Part model, mm, in its own coordinate system. Face numbers are marked on the shaded views. Coordinates: 2 decimals unless noted, no trailing zeros. Order: outer loops, then holes, each group sorted by start corner. A loop starts at its lowest first (then second) coordinate and runs counter-clockwise, first axis right, second up.
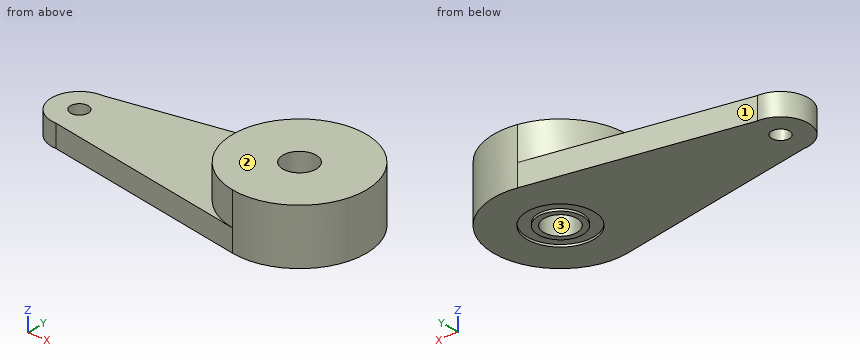
from build123d import *

# Parameters (mm, degrees)
F0_R     = 1.5
F1_DEPTH = 5
F0_R_2   = 0.8
F2_DEPTH = 2
F3_R     = 3
F3_R_2   = 2
F4_DEPTH = 0.2


with BuildPart() as f1:
    # F0 (on Top) → F1 (new body)
    with BuildSketch(Plane.XY):
        with BuildLine():
            ThreePointArc((-1.0798815668, -5.9020213319), (3.8419207826, -4.6086489018), (6, 0))
            ThreePointArc((6, 0), (3.8419207985, 4.6086488886), (-1.0798815261, 5.9020213393))
            ThreePointArc((-1.0798815261, 5.9020213393), (-6, 2.07e-08), (-1.0798815668, -5.9020213319))
        make_face()
        Circle(F0_R, mode=Mode.SUBTRACT)
    extrude(amount=F1_DEPTH)

    # F0 (on Top) → F2 (join)
    with BuildSketch(Plane.XY):
        with BuildLine():
            ThreePointArc((-1.0798815668, -5.9020213319), (-6, 2.07e-08), (-1.0798815261, 5.9020213393))
            Line((-1.0798815261, 5.9020213393), (-19.6734044441, 2.5))
            ThreePointArc((-19.6734044441, 2.5), (-17.9056374912, 1.767766953), (-17.1734044441, 0))
            ThreePointArc((-17.1734044441, 0), (-17.9056374912, -1.767766953), (-19.6734044441, -2.5))
            Line((-19.6734044441, -2.5), (-1.0798815668, -5.9020213319))
        make_face()
        with BuildLine():
            ThreePointArc((-17.1734044441, 0), (-17.9056374912, 1.767766953), (-19.6734044441, 2.5))
            ThreePointArc((-19.6734044441, 2.5), (-22.1734044441, 0), (-19.6734044441, -2.5))
            ThreePointArc((-19.6734044441, -2.5), (-17.9056374912, -1.767766953), (-17.1734044441, 0))
        make_face()
        with Locations((-19.6734044441, 0)):
            Circle(F0_R_2, mode=Mode.SUBTRACT)
    extrude(amount=F2_DEPTH)

    # F3 (on face) → F4 (cut)
    with BuildSketch(Plane(origin=(0, 0, 0), x_dir=(1, 0, 0), z_dir=(0, 0, -1))):
        Circle(F3_R)
        Circle(F3_R_2, mode=Mode.SUBTRACT)
    extrude(amount=-F4_DEPTH, mode=Mode.SUBTRACT)


solid = f1.part
Q1. Wall check: line 1 along Y through (x, z) = (0, 0.1); line 2 along Y through (x, z) = (0, 1.25); line 3 along Z through (x, y) = (-7, 1.25). Give the ranges that are in metal, low to high.
Results list:
line 1: y = -6 to -3, -2 to -1.5, 1.5 to 2, 3 to 6
line 2: y = -6 to -1.5, 1.5 to 6
line 3: z = 0 to 2
Q2. Cut at C-C on y = 0. Write the cut outline in (x, z), and give its area (3 significant figures).
Results list:
outline: (-22.17, 0) - (-20.47, 0) - (-20.47, 2) - (-22.17, 2) - close; (-18.87, 0) - (-3, 0) - (-3, 0.2) - (-2, 0.2) - (-2, 0) - (-1.5, 0) - (-1.5, 5) - (-6, 5) - (-6, 2) - (-18.87, 2) - close; (1.5, 0) - (2, 0) - (2, 0.2) - (3, 0.2) - (3, 0) - (6, 0) - (6, 5) - (1.5, 5) - close
area: 73.7 mm2
Q3. Cut at B-B on z = 1.65. Write the cut outline in (x, y).
Results list:
outline: (-19.67, -2.5) - (-1.08, -5.9) arc R6 ccw (long way) to (-1.08, 5.9) - (-19.67, 2.5) arc R2.5 ccw to start; hole circle Ø1.6 at (-19.67, 0); hole circle Ø3 at (0, 0)
Q4. Cut at A-A on x = 0. Write the cut outline in (y, z).
Results list:
outline: (-6, 0) - (-3, 0) - (-3, 0.2) - (-2, 0.2) - (-2, 0) - (-1.5, 0) - (-1.5, 5) - (-6, 5) - close; (1.5, 0) - (2, 0) - (2, 0.2) - (3, 0.2) - (3, 0) - (6, 0) - (6, 5) - (1.5, 5) - close
Q5. Cut at D-D on z = 2.95. Write the cut outline in (x, y), and give its area (3 significant figures).
Results list:
outline: circle Ø12 at (0, 0); hole circle Ø3 at (0, 0)
area: 106 mm2
Q6. Mould opens along X. For the marked faces 1, 2 and 3 say: pulls with the +X half, pulls with the -X half, needs draft (parallel to the pull), parting line crosses it, or undercut.
Results list:
face 1: pulls with the -X half
face 2: needs draft
face 3: undercut
Q7. Pin check, flat tips, straight feed: pin 1 Ø6 at (x, y) = (-10.5, -0.5) entering from +Z; pin 2 Ø2 at (x, z) = (-4.5, 3.5) entering from +Y; pin 3 Ø1 at (y, z) = (3.5, 4) entering from -X; pin 4 Ø3 at (x, y) = (1, 0) entering from -Z. Stop position of each tip, or through.
Results list:
pin 1: stops at z = 2
pin 2: stops at y = 4.87
pin 3: stops at x = -5.2
pin 4: stops at z = 0
